```python
from build123d import *

# Parameters (mm, degrees)
BOSS_EXTRUDE1_DEPTH      = 6.35
FILLET1_R                = 3.175
M5_CLEARANCE_HOLE1_D     = 5.5
M5_CLEARANCE_HOLE1_DEPTH = 18.75
M5_CLEARANCE_HOLE1_TIP   = 1.652366702


with BuildPart() as part:
    # Sketch1 → Boss-Extrude1 (new body)
    with BuildSketch(Plane.XY):
        Polygon((-12.7, 46.1), (-12.7, 58.239487758), (-43.360512242, 88.9), (-81.460512242, 88.9), (-81.460512242, 114.3), (-32.839487758, 114.3), (9.960512242, 71.5), (12.7, 71.5), (88.9, 71.5), (88.9, 46.1), (12.7, 46.1), (12.7, 20.139487758), (-12.7, 20.139487758), align=None)
    extrude(amount=BOSS_EXTRUDE1_DEPTH)

    # Fillet1
    fillet1_edges = [part.edges().sort_by_distance(p)[0] for p in [
        (-12.7, 58.239487758, 3.175),
        (-43.360512242, 88.9, 3.175),
        (9.960512242, 71.5, 3.175),
        (12.7, 46.1, 3.175),
    ]]
    fillet(fillet1_edges, radius=FILLET1_R)

    # M5 Clearance Hole1
    with Locations(Plane.XY.offset(6.35)):
        with Locations((0, 58.8), (25.4, 58.8), (76.2, 58.8), (-50.8, 101.6), (-68.760512242, 101.6), (0, 32.839487758)):
            Hole(M5_CLEARANCE_HOLE1_D / 2, depth=M5_CLEARANCE_HOLE1_DEPTH)
            with Locations((0, 0, -(M5_CLEARANCE_HOLE1_DEPTH + M5_CLEARANCE_HOLE1_TIP / 2))):  # 118° drill point
                Cone(0, M5_CLEARANCE_HOLE1_D / 2, M5_CLEARANCE_HOLE1_TIP, mode=Mode.SUBTRACT)


solid = part.part
```
Build history of the part. All positions in model axes, mm. A direction names the side the tool comes from. Give positions to 0.01 mm unless a question says otherwise; leave off trailing zeros. Loops run counter-clockwise (first coordinate to the right, second up) from the corner with the lowest first, then second, coordinate; pieces in that order, holes last.
Item 1: Slice it at B-B, the plane z = 1.5. List the corners of the cut face in (x, y) (3 decimals).
Answers follow:
outline: (-81.461, 88.9) - (-44.676, 88.9) arc R3.175 cw to (-42.431, 87.97) - (-13.63, 59.169) arc R3.175 cw to (-12.7, 56.924) - (-12.7, 20.139) - (12.7, 20.139) - (12.7, 42.925) arc R3.175 cw to (15.875, 46.1) - (88.9, 46.1) - (88.9, 71.5) - (11.276, 71.5) arc R3.175 cw to (9.031, 72.43) - (-32.839, 114.3) - (-81.461, 114.3) - close; hole circle Ø5.5 at (-68.761, 101.6); hole circle Ø5.5 at (-50.8, 101.6); hole circle Ø5.5 at (0, 32.839); hole circle Ø5.5 at (0, 58.8); hole circle Ø5.5 at (25.4, 58.8); hole circle Ø5.5 at (76.2, 58.8)
Item 2: Which spindle directions (+Z, -Z, +X, -X, +Y, -Y) get a long thin tool onto all of the face, cutting with end or side? Do faces 1 (the face through (-63, 88.9, 3)), 2 (the face through (-81.461, 101, 3)), 3 (the face through (53, 46.1, 3)). Say none if no direction does.
Answers follow:
face 1: +Z, -Z, -X, -Y
face 2: +Z, -Z, -X, +Y, -Y
face 3: +Z, -Z, +X, -Y
Item 3: Flat gauge pins, fed straight in: pin 1 (1.5 mm diameter, centred on y = 34.5, z = 1.5, fed in from +X); pin 2 (1.5 mm diameter, centred on y = 39.5, z = 2.5, fed in from -X); pin 3 (1.9 mm diameter, centred on x = 52.5, z = 2.5, fed in from -Y). Where does each tip first touch, or does it go through?
Answers follow:
pin 1: stops at x = 12.7
pin 2: stops at x = -12.7
pin 3: stops at y = 46.1
Item 4: Slice it at D-D, the plane x = 0. List the corners of the cut face in (y, z).
Answers follow:
outline: (20.14, 0) - (30.09, 0) - (30.09, 6.35) - (20.14, 6.35) - close; (35.59, 0) - (56.05, 0) - (56.05, 6.35) - (35.59, 6.35) - close; (61.55, 0) - (81.46, 0) - (81.46, 6.35) - (61.55, 6.35) - close
Item 5: Slice it at A-A, the plane x = -50.8. List the corners of the cut face in (y, z), and give its area (3 significant figures).
Answers follow:
outline: (88.9, 0) - (98.85, 0) - (98.85, 6.35) - (88.9, 6.35) - close; (104.35, 0) - (114.3, 0) - (114.3, 6.35) - (104.35, 6.35) - close
area: 126 mm2
Item 6: Slice it at C-C, the plane y = 101.6. List the corners of the cut face in (x, z), and give its area (3 significant figures).
Answers follow:
outline: (-81.46, 0) - (-71.51, 0) - (-71.51, 6.35) - (-81.46, 6.35) - close; (-66.01, 0) - (-53.55, 0) - (-53.55, 6.35) - (-66.01, 6.35) - close; (-48.05, 0) - (-20.14, 0) - (-20.14, 6.35) - (-48.05, 6.35) - close
area: 320 mm2
Item 7: Pull direction Y, two halves, no side cores. Call faces 4 (the face through (0.596, 30.155, 3.131)), 5 (the face through (0, 20.139, 3)), 6 (the face through (-52.07, 99.16, 3.13)), 7 (the face through (88.9, 59, 3)): released by +Y, released by -Y, zero draft, split by the parting line, or undercut.
Answers follow:
face 4: undercut
face 5: released by -Y
face 6: undercut
face 7: zero draft
Item 8: Drill centre lines: line 1 (Y direction, x = 25.4, z = 1.5); line 2 (Y direction, x = 19.5, z = 3.5); line 3 (X direction, y = 48.5, z = 5.5). Where is each one in solid material? Low to high.
Answers follow:
line 1: y = 46.1 to 56.05, 61.55 to 71.5
line 2: y = 46.1 to 71.5
line 3: x = -12.7 to 88.9
